```python
from build123d import *

# Parameters (mm, degrees)
SALIENTE_EXTRUIR1_DEPTH = 25.4
CROQUIS4_R              = 1.5
CROQUIS4_W              = 5.75
CROQUIS4_H              = 12.4
CORTAR_EXTRUIR3_DEPTH   = 29.45013181


with BuildPart() as part:
    # Croquis1 → Saliente-Extruir1 (new body)
    with BuildSketch(Plane.XY):
        with BuildLine():
            Line((0, -2.25), (12, -2.25))
            Line((12, -2.25), (12, -1.25))
            Line((12, -1.25), (1.870828693, -1.25))
            Line((1.870828693, -1.25), (0, -1.25))
            ThreePointArc((0, -1.25), (-0.883883476, 0.883883476), (1.25, 0))
            Line((1.25, 0), (1.25, -0.25))
            Line((1.25, -0.25), (2.236067977, -0.25))
            Line((2.236067977, -0.25), (2.25, -0.25))
            Line((2.25, -0.25), (2.25, 0))
            ThreePointArc((2.25, 0), (-1.590990258, 1.590990258), (0, -2.25))
        make_face()
    extrude(amount=SALIENTE_EXTRUIR1_DEPTH)

    # Croquis4 → Cortar-Extruir3 (cut, through all)
    with BuildSketch(Plane.XZ.offset(2.25)):
        with Locations(Location((8.5, 20.2, 0), (0, 0, 270))):
            Circle(CROQUIS4_R)
        with Locations(Location((8.5, 5.2, 0), (0, 0, 270))):
            Circle(CROQUIS4_R)
        with Locations((0.625, 12.7)):
            Rectangle(CROQUIS4_W, CROQUIS4_H)
    extrude(amount=-CORTAR_EXTRUIR3_DEPTH, mode=Mode.SUBTRACT)


solid = part.part
```
Model file for the job. Use its own axes, mm. A direction names the side the tool comes from. Coordinates: 2 decimals unless noted, no trailing zeros. Loops run counter-clockwise (first coordinate to the right, second up) from the corner with the lowest first, then second, coordinate; pieces in that order, holes last. Notation, with made-up numbers: (16.25, 53) - (71.25, 53) arc R18 cw to (71.25, 68) - close; hole circle Ø10 at (-12.75, 12). An arc over 180 degrees is marked (long way). Answer as a JSON object with one key per item and string values. Group by question number.
(1) Cut at C-C (y = 1.8). Give the cut face in (x, z).
(2) Cut at A-A (z = 20.2). Give the cut face in (x, y).
(3) Tool access for faces 1 (the face through (3.5, -2, 13)), 2 (the face through (7.6, -1.8, 6.4)), 3 (the face through (2, -0.25, 22)): list every direction of +Z, -Z, +X, -X, +Y, -Y with a clear straight run to the whole face (end or side of a thin tool).
(4) Cut at B-B (x = 8.5). Give the cut face in (y, z).
(5) Two-plate mould, pull along Z, no slides. Class faces 4 (the face through (3, -2, 0)), 5 (the face through (-0.913, 0.854, 3.204)), 6 (the face through (0, -2, 18.9)): released by +Z, released by -Z, zero draft, split by the parting line, or undercut.
(6) Probe line 1 along Z through (x, y) = (-1.25, 1.1); line 2 along Y through (x, z) = (0, 21); line 3 along Z through (x, y) = (9.75, -1.85). List the from-to ranges inside material, lowest first.
(7) Flat gauge pins, fed straight in: pin 1 (0.8 mm diameter, centred on y = -2, z = 15, fed in from -X); pin 2 (8 mm diameter, centred on x = 10, z = 4, fed in from +Y). Where does each tip first touch, or does it go through?
(8) Cut at D-D (x = 0.75). Give the cut face in (y, z), then the cut area to 3 significant figures.
Geometry says:
{
 "1": {"outline": "(-1.35, 0) - (1.35, 0) - (1.35, 6.5) - (-1.35, 6.5) - close; (-1.35, 18.9) - (1.35, 18.9) - (1.35, 25.4) - (-1.35, 25.4) - close"},
 "2": {"outline": "(0, -2.25) - (7, -2.25) - (7, -1.25) - (0, -1.25) arc R1.25 cw (long way) to (1.25, 0) - (1.25, -0.25) - (2.25, -0.25) - (2.25, 0) arc R2.25 ccw (long way) to start; (10, -2.25) - (12, -2.25) - (12, -1.25) - (10, -1.25) - close"},
 "3": {"face 1": "-X, +Y, -Y", "face 2": "+Y, -Y", "face 3": "+Z, -Z, +X"},
 "4": {"outline": "(-2.25, 0) - (-1.25, 0) - (-1.25, 3.7) - (-2.25, 3.7) - close; (-2.25, 6.7) - (-1.25, 6.7) - (-1.25, 18.7) - (-2.25, 18.7) - close; (-2.25, 21.7) - (-1.25, 21.7) - (-1.25, 25.4) - (-2.25, 25.4) - close"},
 "5": {"face 4": "released by -Z", "face 5": "zero draft", "face 6": "undercut"},
 "6": {"line 1": "z = 0 to 6.5, 18.9 to 25.4", "line 2": "y = -2.25 to -1.25, 1.25 to 2.25", "line 3": "z = 0 to 4.37, 6.03 to 19.37, 21.03 to 25.4"},
 "7": {"pin 1": "stops at x = 3.5", "pin 2": "stops at y = -1.25"},
 "8": {"outline": "(-2.25, 0) - (-1.25, 0) - (-1.25, 6.5) - (-2.25, 6.5) - close; (-2.25, 18.9) - (-1.25, 18.9) - (-1.25, 25.4) - (-2.25, 25.4) - close; (1, 0) - (2.12, 0) - (2.12, 6.5) - (1, 6.5) - close; (1, 18.9) - (2.12, 18.9) - (2.12, 25.4) - (1, 25.4) - close", "area": "27.6 mm^2"}
}
